from build123d import *

# Parameters (mm, degrees)
PLATE_DEPTH                  = 6.35
D_GAGEMENT_M32_AT_2_COUNT    = 2
D_GAGEMENT_M32_AT_2_PITCH    = 12
D_GAGEMENT_M32_AT_3_COUNT    = 2
D_GAGEMENT_M32_AT_3_PITCH    = 56.568542495
D_GAGEMENT_M32_AT_4_COUNT    = 2
D_GAGEMENT_M32_AT_4_PITCH    = 65.604877867
R_P_TITION_CIRCULAIRE2_COUNT = 4
D_GAGEMENT_M33_D             = 2.6
D_GAGEMENT_M33_DEPTH         = 6.35
D_GAGEMENT_M33_TIP           = 0.781118805
D_GAGEMENT_M51_D             = 4.54
D_GAGEMENT_M51_DEPTH         = 6.35
D_GAGEMENT_M51_TIP           = 1.363953605
BOLTPATTERNPUCK_D            = 2.6
BOLTPATTERNPUCK_DEPTH        = 6.35
BOLTPATTERNPUCK_TIP          = 0.781118805
ENL_V_MAT_EXTRU_1_DEPTH      = 6.35


with BuildPart() as part:
    # Esquisse3 → Plate (new body)
    with BuildSketch(Plane(origin=(0, 0, 0), x_dir=(1, 0, 0), z_dir=(0, 1, 0))):
        Polygon((-54.533236369, 80), (54.533236369, 80), (77.906839173, 29.875147031), (77.906839173, -78.326589525), (50, -155), (-50, -155), (-77.906839173, -78.326589525), (-77.906839173, 29.875147031), align=None)
    extrude(amount=-PLATE_DEPTH)

    # Esquisse10 → Dégagement M32 (revolve, cut)
    with BuildSketch(Plane(origin=(-24, 0, -64), x_dir=(0, 0, 1), z_dir=(1, 0, 0))):
        Polygon((0, 0), (0, 7.31137699), (1.6, 6.35), (1.6, 0), align=None)
    d_gagement_m32 = revolve(axis=Axis((-24, 6.35, -64), (0, -1, 0)), mode=Mode.SUBTRACT)

    # Dégagement M32 at 2: Dégagement M32 ×2
    with Locations(*[(i * D_GAGEMENT_M32_AT_2_PITCH, 0, 0) for i in range(1, D_GAGEMENT_M32_AT_2_COUNT)]):
        add(d_gagement_m32, mode=Mode.SUBTRACT)

    # Dégagement M32 at 3: Dégagement M32 ×2
    with Locations(*[Vector(-0.7071067811865476, 0, 0.7071067811865475) * (i * D_GAGEMENT_M32_AT_3_PITCH) for i in range(1, D_GAGEMENT_M32_AT_3_COUNT)]):
        add(d_gagement_m32, mode=Mode.SUBTRACT)

    # Dégagement M32 at 4: Dégagement M32 ×2
    with Locations(*[Vector(-0.6097107608496924, 0, 0.7926239891046001) * (i * D_GAGEMENT_M32_AT_4_PITCH) for i in range(1, D_GAGEMENT_M32_AT_4_COUNT)]):
        add(d_gagement_m32, mode=Mode.SUBTRACT)

    # Répétition circulaire2: Dégagement M32 ×4 about axis
    r_p_tition_circulaire2_axis = Axis((0, 0, 0), (0, 1, 0))
    for i in range(1, R_P_TITION_CIRCULAIRE2_COUNT):
        add(d_gagement_m32.rotate(r_p_tition_circulaire2_axis, i * 360 / R_P_TITION_CIRCULAIRE2_COUNT), mode=Mode.SUBTRACT)

    # Répétition circulaire2 copy 1 sketch → Répétition circulaire2 copy 1 (revolve, cut)
    with BuildSketch(Plane(origin=(-64, 0, 12), x_dir=(1, 0, 0), z_dir=(0, 0, -1))):
        Polygon((0, 0), (0, 7.31137699), (1.6, 6.35), (1.6, 0), align=None)
    revolve(axis=Axis((-64, 6.35, 12), (0, -1, 0)), mode=Mode.SUBTRACT)

    # Répétition circulaire2 copy 2 sketch → Répétition circulaire2 copy 2 (revolve, cut)
    with BuildSketch(Plane(origin=(12, 0, 64), x_dir=(0, 0, -1), z_dir=(-1, 0, 0))):
        Polygon((0, 0), (0, 7.31137699), (1.6, 6.35), (1.6, 0), align=None)
    revolve(axis=Axis((12, 6.35, 64), (0, -1, 0)), mode=Mode.SUBTRACT)

    # Répétition circulaire2 copy 3 sketch → Répétition circulaire2 copy 3 (revolve, cut)
    with BuildSketch(Plane(origin=(64, 0, -12), x_dir=(-1, 0, 0), z_dir=(0, 0, 1))):
        Polygon((0, 0), (0, 7.31137699), (1.6, 6.35), (1.6, 0), align=None)
    revolve(axis=Axis((64, 6.35, -12), (0, -1, 0)), mode=Mode.SUBTRACT)

    # Répétition circulaire2 copy 4 sketch → Répétition circulaire2 copy 4 (revolve, cut)
    with BuildSketch(Plane(origin=(-24, 0, 64), x_dir=(1, 0, 0), z_dir=(0, 0, -1))):
        Polygon((0, 0), (0, 7.31137699), (1.6, 6.35), (1.6, 0), align=None)
    revolve(axis=Axis((-24, 6.35, 64), (0, -1, 0)), mode=Mode.SUBTRACT)

    # Répétition circulaire2 copy 5 sketch → Répétition circulaire2 copy 5 (revolve, cut)
    with BuildSketch(Plane(origin=(64, 0, 24), x_dir=(0, 0, -1), z_dir=(-1, 0, 0))):
        Polygon((0, 0), (0, 7.31137699), (1.6, 6.35), (1.6, 0), align=None)
    revolve(axis=Axis((64, 6.35, 24), (0, -1, 0)), mode=Mode.SUBTRACT)

    # Répétition circulaire2 copy 6 sketch → Répétition circulaire2 copy 6 (revolve, cut)
    with BuildSketch(Plane(origin=(24, 0, -64), x_dir=(-1, 0, 0), z_dir=(0, 0, 1))):
        Polygon((0, 0), (0, 7.31137699), (1.6, 6.35), (1.6, 0), align=None)
    revolve(axis=Axis((24, 6.35, -64), (0, -1, 0)), mode=Mode.SUBTRACT)

    # Répétition circulaire2 copy 7 sketch → Répétition circulaire2 copy 7 (revolve, cut)
    with BuildSketch(Plane(origin=(-12, 0, 64), x_dir=(1, 0, 0), z_dir=(0, 0, -1))):
        Polygon((0, 0), (0, 7.31137699), (1.6, 6.35), (1.6, 0), align=None)
    revolve(axis=Axis((-12, 6.35, 64), (0, -1, 0)), mode=Mode.SUBTRACT)

    # Répétition circulaire2 copy 8 sketch → Répétition circulaire2 copy 8 (revolve, cut)
    with BuildSketch(Plane(origin=(64, 0, 12), x_dir=(0, 0, -1), z_dir=(-1, 0, 0))):
        Polygon((0, 0), (0, 7.31137699), (1.6, 6.35), (1.6, 0), align=None)
    revolve(axis=Axis((64, 6.35, 12), (0, -1, 0)), mode=Mode.SUBTRACT)

    # Répétition circulaire2 copy 9 sketch → Répétition circulaire2 copy 9 (revolve, cut)
    with BuildSketch(Plane(origin=(12, 0, -64), x_dir=(-1, 0, 0), z_dir=(0, 0, 1))):
        Polygon((0, 0), (0, 7.31137699), (1.6, 6.35), (1.6, 0), align=None)
    revolve(axis=Axis((12, 6.35, -64), (0, -1, 0)), mode=Mode.SUBTRACT)

    # Dégagement M33
    with Locations(Plane(origin=(0, 0, 0), x_dir=(1, 0, 0), z_dir=(0, 1, 0))):
        with Locations((13.379268261, 74.387466557), (-64.260298072, 39.788366286), (-13.379268261, -74.387466557), (64.260298072, -39.788366286)):
            Hole(D_GAGEMENT_M33_D / 2, depth=D_GAGEMENT_M33_DEPTH)
            with Locations((0, 0, -(D_GAGEMENT_M33_DEPTH + D_GAGEMENT_M33_TIP / 2))):  # 118° drill point
                Cone(0, D_GAGEMENT_M33_D / 2, D_GAGEMENT_M33_TIP, mode=Mode.SUBTRACT)

    # Dégagement M51
    with Locations(Plane(origin=(0, 0, 0), x_dir=(1, 0, 0), z_dir=(0, 1, 0))):
        with Locations((-27.48, -118), (27.48, -118)):
            Hole(D_GAGEMENT_M51_D / 2, depth=D_GAGEMENT_M51_DEPTH)
            with Locations((0, 0, -(D_GAGEMENT_M51_DEPTH + D_GAGEMENT_M51_TIP / 2))):  # 118° drill point
                Cone(0, D_GAGEMENT_M51_D / 2, D_GAGEMENT_M51_TIP, mode=Mode.SUBTRACT)

    # BoltPatternPuck
    with Locations(Plane(origin=(-22.655, 0, 88.899176296), x_dir=(0, 0, 1), z_dir=(0, 1, 0))):
        with Locations((0, 0), (0, 45.31)):
            Hole(BOLTPATTERNPUCK_D / 2, depth=BOLTPATTERNPUCK_DEPTH)
            with Locations((0, 0, -(BOLTPATTERNPUCK_DEPTH + BOLTPATTERNPUCK_TIP / 2))):  # 118° drill point
                Cone(0, BOLTPATTERNPUCK_D / 2, BOLTPATTERNPUCK_TIP, mode=Mode.SUBTRACT)

    # Esquisse19 → Enlèv. mat.-Extru.1 (cut)
    with BuildSketch(Plane(origin=(0, 0, 0), x_dir=(1, 0, 0), z_dir=(0, 1, 0))):
        with BuildLine():
            Line((20.271956718, -59.39121964), (56.808223228, -43.1092901))
            ThreePointArc((56.808223228, -43.1092901), (68.032089888, -47.413336706), (63.728043282, -58.637203367))
            Line((63.728043282, -58.637203367), (27.191776772, -74.919132906))
            ThreePointArc((27.191776772, -74.919132906), (15.967910112, -70.6150863), (20.271956718, -59.39121964))
        make_face()
        with BuildLine():
            Line((-46.588263316, -40.402999759), (-30.306333777, -76.939266269))
            ThreePointArc((-30.306333777, -76.939266269), (-34.610380383, -88.163132929), (-45.834247043, -83.859086323))
            Line((-45.834247043, -83.859086323), (-62.116176583, -47.322819813))
            ThreePointArc((-62.116176583, -47.322819813), (-57.812129976, -36.098953153), (-46.588263316, -40.402999759))
        make_face()
    extrude(amount=-ENL_V_MAT_EXTRU_1_DEPTH, mode=Mode.SUBTRACT)


solid = part.part
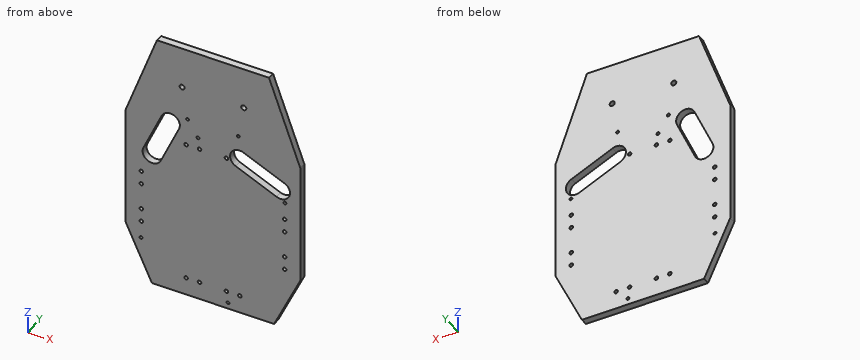
CAD build for the part. Positions are in the model's coordinates, mm. Give positions to 0.01 mm unless a question says otherwise; leave off trailing zeros. Loops run counter-clockwise (first coordinate to the right, second up) from the corner with the lowest first, then second, coordinate; pieces in that order, holes last. Notation, with made-up numbers: M 58.5,6 L 91.5,6 A26 cw 91.5,34 Z; hole C 61,-16.5 d4. An arc over 180 degrees is marked long. One line per question, with ' | ' between items. Start each with the question number.
1. Saw through at C-C on z = -44. Give the cut face in (x, y), plus the area to 3 significant figures.
2. Flat gauge pins, fed straight in: pin 1 (4 mm diameter, centred on x = -64, z = 24, fed in from +Y); pin 2 (1.9 mm diameter, centred on x = 64, z = -12, fed in from +Y). Where does each tip first touch, or does it go through?
3. Saw through at B-B on y = -3.25. State how many separate pieces and enclosed holes the cut face has, plus the area to 3 significant figures.
4. Saw through at A-A on x = -42.5. Give the cut face in (y, z), plus the area to 3 significant figures.
5. Probe L1, parallel to Z at x = -24, y = -5; L2, parallel to X at y = -2.5, z = 24; L3, parallel to X at y = -1.5, z = 64.5. List the from-to ranges inside material, lowest first. Write a range as from..to.
Result sheet:
1) outline: M -71.32,-6.35 L 71.32,-6.35 L 71.32,0 L -71.32,0 Z | area: 906 mm^2
2) pin 1: stops at y = 0 | pin 2: passes through
3) separate pieces: 1 | enclosed holes: 25 | area: 31,300 mm^2
4) outline: M -6.35,-80 L 0,-80 L 0,49.58 L -6.35,49.58 Z; M -6.35,87.65 L 0,87.65 L 0,155 L -6.35,155 Z | area: 1,250 mm^2
5) L1: z = -80..-65.6, -62.4..62.4, 65.6..155 | L2: x = -77.91..-65.6, -62.4..62.4, 65.6..77.91 | L3: x = -77.91..-54.46, -35.85..-25.52, -22.48..-13.52, -10.48..10.48, 13.52..15.66, 50.57..77.91
